The drawing under review shows one solid part. Ordinate dimensions are in mm from its lowest x, y, z. A direction names the side the tool comes from. Give positions to 0.01 mm unless a question says otherwise; leave off trailing zeros. Write each loop counter-clockwise with the first axis right and the second up, starting at its lowest first coordinate (ties: lowest second). Pieces come first, ordered by that corner, then holes.
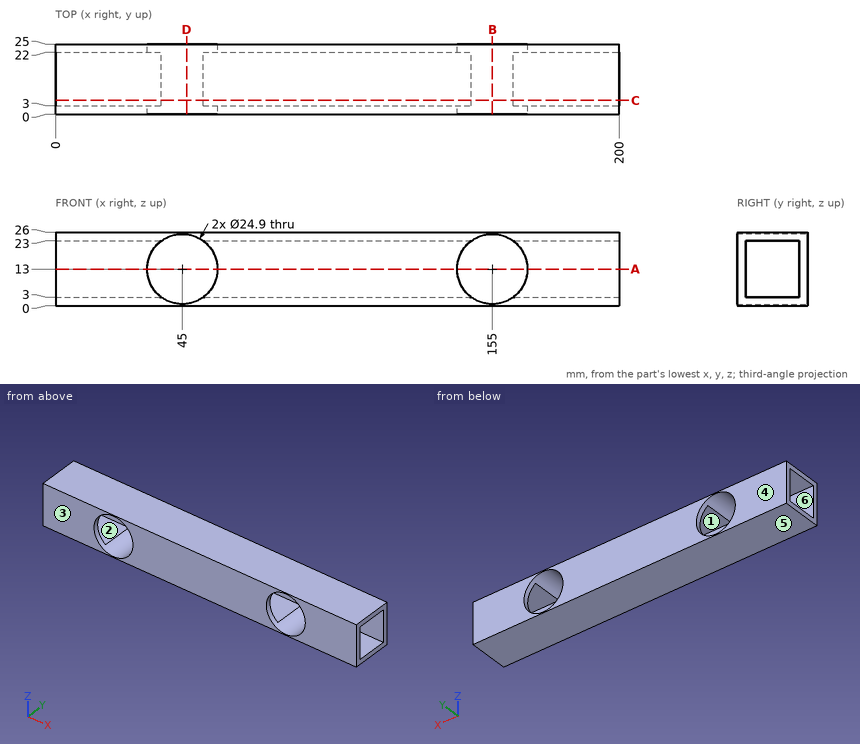
1) Consider section C-C, the plane y = 5. Give the boundary of the cut face in (x, z).
2) Consider section A-A, the plane z = 13. Give the boundary of the cut face in (x, y).
3) Tool access review of the marked faces 5 and 6: name each direction out of +Z, -Z, +X, -X, +Y, -Y from which nothing blocks a thin tool from reaching the whole face with its end or side.
4) Consider section D-D, the plane x = 46.5. Give the boundary of the cut face in (y, z), then the cut area to 3 significant figures.
5) The part is to be moulded in two halves that separate along Y. For the marked faces 1, 2, 3 and 4, say which applies: +Y half, -Y half, draft (parallel to the pull), parting line (faces both ways), or undercut.
6) Insertion check: pin 1 (15 mm diameter, centred on x = 155, z = 13, fed in from +Y). The pin has a flat end and moves straight along its axis. Give the tip position at first contact, or say it passes through.
7) To check wall thickness, follow probe 1 along Z at (x, y) = (132.5, 17.25); probe 2 along Z at (x, y) = (45, 9.5); probe 3 along Y at (x, z) = (60, 11.5). State the ranges of each line that lie inside material, in increasing order.
8) Consider section B-B, the plane x = 155. Give the boundary of the cut face in (y, z).
Answer block:
1. outline: (0, 0) - (200, 0) - (200, 3) - (162.42, 3) arc R12.45 cw to (147.58, 3) - (52.42, 3) arc R12.45 cw to (37.58, 3) - (0, 3) - close; (0, 23) - (37.58, 23) arc R12.45 cw to (52.42, 23) - (147.58, 23) arc R12.45 cw to (162.42, 23) - (200, 23) - (200, 26) - (0, 26) - close
2. outline: (0, 0) - (32.55, 0) - (32.55, 3) - (0, 3) - close; (0, 22) - (32.55, 22) - (32.55, 25) - (0, 25) - close; (57.45, 0) - (142.55, 0) - (142.55, 3) - (57.45, 3) - close; (57.45, 22) - (142.55, 22) - (142.55, 25) - (57.45, 25) - close; (167.45, 0) - (200, 0) - (200, 3) - (167.45, 3) - close; (167.45, 22) - (200, 22) - (200, 25) - (167.45, 25) - close
3. face 5: -Z, +X, -X, +Y, -Y
3. face 6: +X, -X
4. outline: (0, 0) - (25, 0) - (25, 0.64) - (0, 0.64) - close; (0, 25.36) - (25, 25.36) - (25, 26) - (0, 26) - close
4. area: 32.0 mm2
5. face 1: undercut
5. face 2: undercut
5. face 3: -Y half
5. face 4: +Y half
6. pin 1: passes through
7. probe 1: z = 0 to 3, 23 to 26
7. probe 2: z = 0 to 0.55, 25.45 to 26
7. probe 3: y = 0 to 3, 22 to 25
8. outline: (0, 0) - (25, 0) - (25, 0.55) - (0, 0.55) - close; (0, 25.45) - (25, 25.45) - (25, 26) - (0, 26) - close
